from build123d import *

# Parameters (mm, degrees)
SKETCH1_W            = 120
SKETCH1_H            = 90
PLATE_DEPTH          = 4
SLOT_CUT_DEPTH       = 76.106590923
SECOND_SLOT_COUNT    = 2
SECOND_SLOT_PITCH    = 13.38
MOTOR_OUTLINE_R      = 1.2
MOTOR_MOUNT_DEPTH    = 76.106590923
MOTORS_COUNT         = 3
MOTORS_PITCH         = 39
MOTORS_COUNT_DIR2    = 2
MOTORS_PITCH_DIR2    = 23
MOTOR_CUTOUT_DEPTH   = 76.106590923
CUTOUT_PATTERN_COUNT = 3
CUTOUT_PATTERN_PITCH = 39
FILLET1_R            = 10
SKETCH5_W            = 28
SKETCH5_H            = 2.3
BOSS_EXTRUDE1_DEPTH  = 4
SKETCH6_W            = 40.5
SKETCH6_H            = 39.62
CUT_EXTRUDE1_DEPTH   = 76.106590923
U2D2_MOUNT_DEPTH     = 76.106590923
BOSS_EXTRUDE2_DEPTH  = 4
THUMB_MOUNT_DEPTH    = 76.106590923
FILLET3_R            = 7


with BuildPart() as part:
    # Sketch1 → plate (new body)
    with BuildSketch(Plane.XY):
        Rectangle(SKETCH1_W, SKETCH1_H)
    extrude(amount=PLATE_DEPTH)

    # Sketch2 → slot_cut (cut, through all)
    with BuildSketch(Plane.XY.offset(4)):
        with BuildLine():
            Line((50, 36.8), (-50, 36.8))
            ThreePointArc((-50, 36.8), (-51.6, 38.4), (-50, 40))
            Line((-50, 40), (50, 40))
            ThreePointArc((50, 40), (51.6, 38.4), (50, 36.8))
        make_face()
    slot_cut = extrude(amount=-SLOT_CUT_DEPTH, mode=Mode.SUBTRACT)

    # second_slot: slot_cut ×2
    with Locations(*[(0, -i * SECOND_SLOT_PITCH, 0) for i in range(1, SECOND_SLOT_COUNT)]):
        add(slot_cut, mode=Mode.SUBTRACT)

    # motor_outline → motor_mount (cut, through all)
    with BuildSketch(Plane.XY.offset(4)):
        with Locations((-54, 16.42)):
            Circle(MOTOR_OUTLINE_R)
        with Locations(Location((-54, 0.42, 0), (0, 0, 180))):
            Circle(MOTOR_OUTLINE_R)
        with Locations((-24, 0.42)):
            Circle(MOTOR_OUTLINE_R)
        with Locations(Location((-24, 16.42, 0), (0, 0, 180))):
            Circle(MOTOR_OUTLINE_R)
    motor_mount = extrude(amount=-MOTOR_MOUNT_DEPTH, mode=Mode.SUBTRACT)

    # motors: motor_mount 3 × 2
    with Locations(*[(i * MOTORS_PITCH, -j * MOTORS_PITCH_DIR2, 0) for i in range(MOTORS_COUNT) for j in range(MOTORS_COUNT_DIR2) if (i, j) != (0, 0)]):
        add(motor_mount, mode=Mode.SUBTRACT)

    # motor_outline<5> → motor_cutout (cut, through all)
    with BuildSketch(Plane.XY.offset(4)):
        with BuildLine():
            Line((-26, -30), (-26, -1.58))
            Line((-26, -1.58), (-52, -1.58))
            Line((-52, -1.58), (-52, -30))
            ThreePointArc((-52, -30), (-50.535533906, -33.535533906), (-47, -35))
            Line((-47, -35), (-31, -35))
            ThreePointArc((-31, -35), (-27.464466094, -33.535533906), (-26, -30))
        make_face()
        with BuildLine():
            Line((-52, -1.58), (-26, -1.58))
            Line((-26, -1.58), (-26, 16.42))
            ThreePointArc((-26, 16.42), (-26.105468435, 17.441548218), (-26.417424305, 18.42))
            Line((-26.417424305, 18.42), (-51.582575695, 18.42))
            ThreePointArc((-51.582575695, 18.42), (-51.894531565, 17.441548218), (-52, 16.42))
            Line((-52, 16.42), (-52, -1.58))
        make_face()
        with BuildLine():
            Line((-51.582575695, 18.42), (-26.417424305, 18.42))
            ThreePointArc((-26.417424305, 18.42), (-28.261387212, 20.603300133), (-31, 21.42))
            Line((-31, 21.42), (-47, 21.42))
            ThreePointArc((-47, 21.42), (-49.738612788, 20.603300133), (-51.582575695, 18.42))
        make_face()
    motor_cutout = extrude(amount=-MOTOR_CUTOUT_DEPTH, mode=Mode.SUBTRACT)

    # cutout_pattern: motor_cutout ×3
    with Locations(*[(i * CUTOUT_PATTERN_PITCH, 0, 0) for i in range(1, CUTOUT_PATTERN_COUNT)]):
        add(motor_cutout, mode=Mode.SUBTRACT)

    # Fillet1
    fillet1_edges = [part.edges().sort_by_distance(p)[0] for p in [
        (-60, 45, 2),
        (60, 45, 2),
    ]]
    fillet(fillet1_edges, radius=FILLET1_R)

    # Sketch5 → Boss-Extrude1 (add)
    with BuildSketch(Plane.XY.offset(4)):
        with Locations((38, -4.23)):
            Rectangle(SKETCH5_W, SKETCH5_H)
    extrude(amount=-BOSS_EXTRUDE1_DEPTH)

    # Sketch6 → Cut-Extrude1 (cut, through all)
    with BuildSketch(Plane.XY.offset(4)):
        with Locations((39.75, -25.19)):
            Rectangle(SKETCH6_W, SKETCH6_H)
    extrude(amount=-CUT_EXTRUDE1_DEPTH, mode=Mode.SUBTRACT)

    # Sketch7 → U2D2_mount (cut, through all)
    with BuildSketch(Plane.XY.offset(4)):
        with BuildLine():
            Line((-50, -38), (8, -38))
            ThreePointArc((8, -38), (9.6, -39.6), (8, -41.2))
            Line((8, -41.2), (-50, -41.2))
            ThreePointArc((-50, -41.2), (-51.6, -39.6), (-50, -38))
        make_face()
    extrude(amount=-U2D2_MOUNT_DEPTH, mode=Mode.SUBTRACT)

    # Sketch8 → Boss-Extrude2 (add)
    with BuildSketch(Plane.XY.offset(4)):
        Polygon((19.5, -5.38), (60, -5.38), (60, -12.38), (26.5, -12.38), (26.5, -45), (19.5, -45), align=None)
    extrude(amount=-BOSS_EXTRUDE2_DEPTH)

    # Sketch9 → thumb_mount (cut, through all)
    with BuildSketch(Plane.XY.offset(4)):
        with BuildLine():
            Line((30, -6.13), (55, -6.13))
            ThreePointArc((55, -6.13), (56.6, -7.73), (55, -9.33))
            Line((55, -9.33), (30, -9.33))
            ThreePointArc((30, -9.33), (28.4, -7.73), (30, -6.13))
        make_face()
        with BuildLine():
            Line((22.5, -15), (22.5, -40))
            ThreePointArc((22.5, -40), (20.9, -41.6), (19.3, -40))
            Line((19.3, -40), (19.3, -15))
            ThreePointArc((19.3, -15), (20.9, -13.4), (22.5, -15))
        make_face()
    extrude(amount=-THUMB_MOUNT_DEPTH, mode=Mode.SUBTRACT)

    # Fillet3
    fillet3_edges = [part.edges().sort_by_distance(p)[0] for p in [
        (60, -12.38, 2),
        (26.5, -12.38, 2),
        (26.5, -45, 2),
        (-60, -45, 2),
    ]]
    fillet(fillet3_edges, radius=FILLET3_R)


solid = part.part
For this review, take the finished solid that the model builds, in its own axes (mm). A direction names the side the tool comes from. Give positions to 0.01 mm unless a question says otherwise; leave off trailing zeros. Write each loop counter-clockwise with the first axis right and the second up, starting at its lowest first coordinate (ties: lowest second). Pieces come first, ordered by that corner, then holes. Notation, with made-up numbers: (41, 26) -> (93, 26) arc R20 cw to (93, 55) -> close; hole circle Ø2 at (35.5, 77.25). An arc over 180 degrees is marked (long way). Use CSV: the item, a comma, the result in double quotes.
Q1. Take a section at B-B, the plane x = 0. Write out the cut boundary in (y, z).
Conclusion:
outline,"(-45, 0) -> (-41.2, 0) -> (-41.2, 4) -> (-45, 4) -> close; (-38, 0) -> (-35, 0) -> (-35, 4) -> (-38, 4) -> close; (21.42, 0) -> (23.42, 0) -> (23.42, 4) -> (21.42, 4) -> close; (26.62, 0) -> (36.8, 0) -> (36.8, 4) -> (26.62, 4) -> close; (40, 0) -> (45, 0) -> (45, 4) -> (40, 4) -> close"
Q2. For P1, Ø3, axis at x = 15, y = 0.42, coming from the +Z side; P2, Ø1.4, axis at x = -54, y = 0.42, coming from the +Z side, all flat-tipped, find the tip position at first contact; note any pin that passes through.
Conclusion:
P1,"z = 4"
P2,"through"
Q3. Take a section at D-D, the plane z = 2.45. State how many separate pieces and enclosed holes the cut face has, then the cut area to 3 significant figures.
Conclusion:
separate pieces,"1"
enclosed holes,"28"
area,"5,010 mm2"
Q4. Mouldability with a two-part tool opening along Y and no side actions: class faces 1 (the face through (-52, -6, 2)), 2 (the face through (24.5, -42.9, 2)) as pulls with the +Y half, pulls with the -Y half, needs draft (parallel to the pull), parting line crosses it, or undercut.
Conclusion:
face 1,"undercut"
face 2,"pulls with the -Y half"
Q5. Take a section at A-A, the plane y = 5.5. Write out the cut boundary in (x, z), then the cut area to 3 significant figures.
Conclusion:
outline,"(-60, 0) -> (-52, 0) -> (-52, 4) -> (-60, 4) -> close; (-26, 0) -> (-13, 0) -> (-13, 4) -> (-26, 4) -> close; (13, 0) -> (26, 0) -> (26, 4) -> (13, 4) -> close; (52, 0) -> (60, 0) -> (60, 4) -> (52, 4) -> close"
area,"168 mm2"
Q6. Take a section at C-C, the plane y = 38.4. Write out the cut boundary in (x, z).
Conclusion:
outline,"(-59.4, 0) -> (-51.6, 0) -> (-51.6, 4) -> (-59.4, 4) -> close; (51.6, 0) -> (59.4, 0) -> (59.4, 4) -> (51.6, 4) -> close"
Q7. To check wall thickness, follow probe 1 along X at (y, z) = (-29.5, 3.8); probe 2 along Y at (x, z) = (41, 0.4); probe 3 along Y at (x, z) = (-18, 0.25). State the ranges of each line that lie inside material, in increasing order. Write a range as [from, to].
Conclusion:
probe 1,"[-60, -52], [-26, -13], [13, 19.3], [22.5, 26.5]"
probe 2,"[-12.38, -9.33], [-6.13, -3.08], [21.42, 23.42], [26.62, 36.8], [40, 45]"
probe 3,"[-45, -41.2], [-38, 23.42], [26.62, 36.8], [40, 45]"
Q8. Tool access review of faces 3 (the face through (-51, -33, 2)), 4 (the face through (-16, -45, 2)): name each direction out of +Z, -Z, +X, -X, +Y, -Y from which nothing blocks a thin tool from reaching the whole face with its end or side.
Conclusion:
face 3,"+Z, -Z"
face 4,"+Z, -Z, +X, -X, -Y"
